Design review of the part built by this model. Coordinates are the model's own, in mm. Round coordinates to 2 decimals unless told otherwise and drop trailing zeros. Write each loop counter-clockwise with the first axis right and the second up, starting at its lowest first coordinate (ties: lowest second). Pieces come first, ordered by that corner, then holes. Notation, with made-up numbers: (-22, 3.25) - (-1, 3.25) arc R9 ccw to (-1, 7.25) - close; hole circle Ø7 at (56.25, 26.5). An arc over 180 degrees is marked (long way). Use one line per item in the form item = value.
```python
from build123d import *

# Parameters (mm, degrees)
F1_DEPTH = 15
F2_R     = 9
F3_DEPTH = 18


with BuildPart() as f1:
    # F0 (on Top) → F1 (new body)
    with BuildSketch(Plane.XY):
        Polygon((-5.802325, -25.549469), (22.505972, -13.413559), (19.711781, 17.259434), (-10.323421, 24.080476), (-26.092006, -2.376881), align=None)
    extrude(amount=F1_DEPTH)

    # F2 (on face) → F3 (cut)
    with BuildSketch(Plane.XY.offset(15)):
        Circle(F2_R)
    extrude(amount=-F3_DEPTH, mode=Mode.SUBTRACT)


solid = f1.part
```
Q1. We need section B-B on y = 0. Write out the cut boundary in (x, z).
Calculated:
outline = (-24.68, 0) - (-9, 0) - (-9, 15) - (-24.68, 15) - close; (9, 0) - (21.28, 0) - (21.28, 15) - (9, 15) - close
Q2. To check wall thickness, follow line 1 along X through (y, z) = (1, 13); line 2 along X through (y, z) = (4.5, 12.5); line 3 along Y through (x, z) = (0, 9.5). State the ranges of each line that lie inside material, in increasing order. Write a range as from..to.
Calculated:
line_1 = -24.08..-8.94, 8.94..21.19
line_2 = -21.99..-7.79, 7.79..20.87
line_3 = -23.06..-9, 9..21.74
Q3. For P1, Ø8, axis at x = 9.5, z = 9, coming from the +Y side; P2, Ø1, axis at x = 12.5, z = 4, coming from the -Y side; P3, Ø1.5, axis at x = -6.5, z = 3.5, coming from the -Y side; P4, Ø8, axis at x = -4.5, z = 10.5, coming from the +Y side, all flat-tipped, find the tip position at first contact; note any pin that passes through.
Calculated:
P1 = 20.49
P2 = -17.92
P3 = -25.55
P4 = 23.67
Q4. Draft analysis for pull direction X (two halves, no side actions). For faces 1 (the flat face through (-8, 5, 0)), 2 (the cylindrical face through (-1.172, 8.923, 7.605)), 3 (the flat face through (4.904, 20.622, 7.395)), state which applies: released by +X, released by -X, zero draft, split by the parting line, or undercut.
Calculated:
face_1 = zero draft
face_2 = undercut
face_3 = released by +X
Q5. We need section A-A on z = 7.25. Write out the cut boundary in (x, y), then the cut area to 3 significant figures.
Calculated:
outline = (-26.09, -2.38) - (-5.8, -25.55) - (22.51, -13.41) - (19.71, 17.26) - (-10.32, 24.08) - close; hole circle Ø18 at (0, 0)
area = 1,380 mm2
Q6. We need section D-D on y = 10. Write out the cut boundary in (x, z), then the cut area to 3 significant figures.
Calculated:
outline = (-18.72, 0) - (20.37, 0) - (20.37, 15) - (-18.72, 15) - close
area = 586 mm2
Q7. We need section C-C on x = 3. Write out the cut boundary in (y, z), then the cut area to 3 significant figures.
Calculated:
outline = (-21.78, 0) - (-8.49, 0) - (-8.49, 15) - (-21.78, 15) - close; (8.49, 0) - (21.05, 0) - (21.05, 15) - (8.49, 15) - close
area = 388 mm2
